The drawing under review shows one solid part. Ordinate dimensions are in mm from its lowest x, y, z. A direction names the side the tool comes from. Round coordinates to 2 decimals unless told otherwise and drop trailing zeros. Write each loop counter-clockwise with the first axis right and the second up, starting at its lowest first coordinate (ties: lowest second). Pieces come first, ordered by that corner, then holes.
Item 1: Add section D-D (z = 7). State how many separate pieces and enclosed holes the cut face has, plus the area to 3 significant figures.
Item 2: Add section A-A (x = 37). Give the boundary of the cut face in (y, z), plus the area to 3 significant figures.
Item 3: Draft analysis for pull direction X (two halves, no side actions). For the marked faces 5, 6, 7 and 8, state which applies: +X half, -X half, draft (parallel to the pull), parting line (faces both ways), or undercut.
Item 4: Add section B-B (y = 27.8). Give the boundary of the cut face in (x, z), plus the area to 3 significant figures.
Item 5: Machinability: for the marked faces 1, 2, 3 and 4, which of the approach directions +Z, -Z, +X, -X, +Y, -Y give a long, thin tool a straight path to every point of the face, cutting with its end or side? Answer none if there is none.
Item 6: Clearance check with flat-ended pins moving along their axes: pin 1 Ø3.5 at (x, z) = (5, 7) entering from -Y; pin 2 Ø10 at (x, y) = (5, 7) entering from -Z; pin 3 Ø3.5 at (y, z) = (28.5, 8) entering from -X; pin 4 Ø1.5 at (x, z) = (36, 10.5) entering from +Y. State where each tip first meets the part, or that it passes through.
Item 7: To check wall thickness, follow L1, parallel to Y at x = 27.5, z = 7; L2, parallel to X at y = 30, z = 2.25; L3, parallel to X at y = 20, z = 7.75. State the ranges of each line that lie inside material, in increasing order.
Item 8: Add section C-C (y = 20). Give the boundary of the cut face in (x, z), plus the area to 3 significant figures.
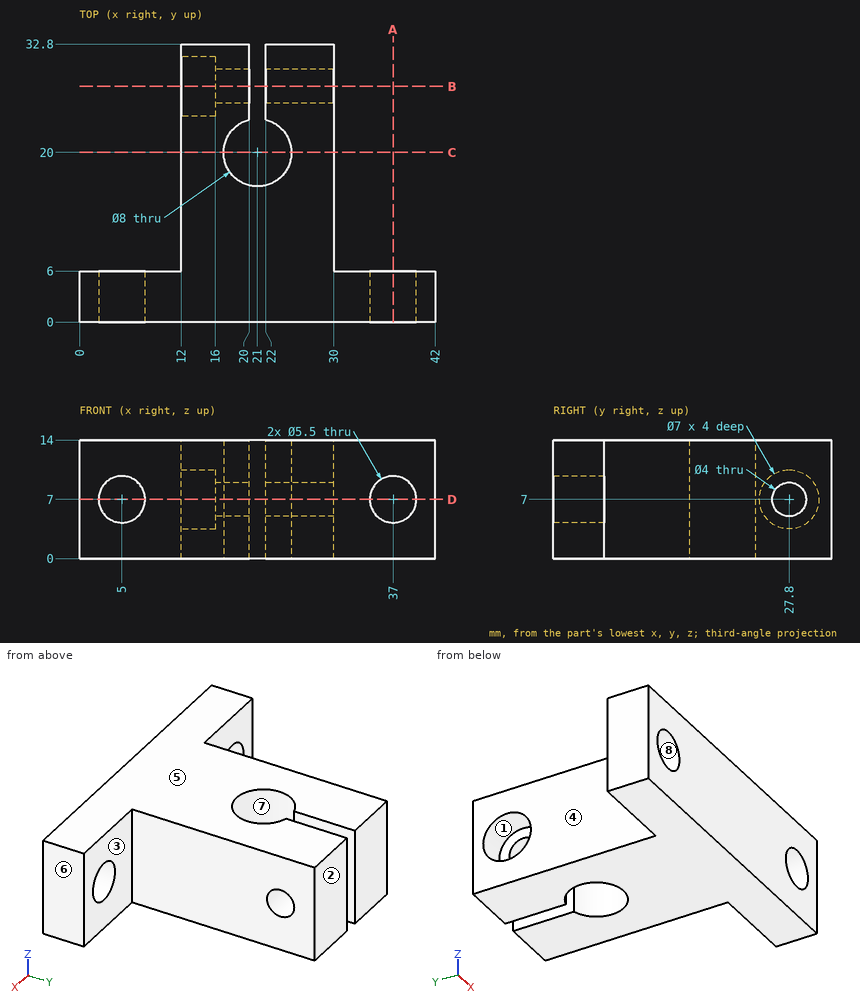
Numbers:
1. separate pieces: 5
1. enclosed holes: 0
1. area: 524 mm2
2. outline: (0, 0) - (6, 0) - (6, 4.25) - (0, 4.25) - close; (0, 9.75) - (6, 9.75) - (6, 14) - (0, 14) - close
2. area: 51.0 mm2
3. face 5: draft
3. face 6: +X half
3. face 7: undercut
3. face 8: undercut
4. outline: (12, 0) - (20, 0) - (20, 5) - (16, 5) - (16, 3.5) - (12, 3.5) - close; (12, 10.5) - (16, 10.5) - (16, 9) - (20, 9) - (20, 14) - (12, 14) - close; (22, 0) - (30, 0) - (30, 5) - (22, 5) - close; (22, 9) - (30, 9) - (30, 14) - (22, 14) - close
4. area: 148 mm2
5. face 1: -X
5. face 2: +Z, -Z, +X, -X, +Y
5. face 3: +Z, -Z, +X, +Y
5. face 4: +Z, -Z, -X, +Y
6. pin 1: passes through
6. pin 2: stops at z = 0
6. pin 3: stops at x = 16
6. pin 4: stops at y = 6
7. L1: y = 0 to 25.8, 29.8 to 32.8
7. L2: x = 12 to 20, 22 to 30
7. L3: x = 12 to 17, 25 to 30
8. outline: (12, 0) - (17, 0) - (17, 14) - (12, 14) - close; (25, 0) - (30, 0) - (30, 14) - (25, 14) - close
8. area: 140 mm2
